from build123d import *

# Parameters (mm, degrees)
SKETCH1_R           = 1.5
SKETCH1_R_2         = 3.5
BOSS_EXTRUDE1_DEPTH = 5
FILLET1_R           = 3
FILLET2_R           = 8
SKETCH2_R           = 3.5
CUT_EXTRUDE1_DEPTH  = 2.5
CUT_EXTRUDE2_DEPTH  = 2


with BuildPart() as part:
    # Sketch1 → Boss-Extrude1 (new body)
    with BuildSketch(Plane(origin=(0, 0, 0), x_dir=(1, 0, 0), z_dir=(0, 1, 0))):
        Polygon((-34, -43.5), (-34, 43.5), (-97, 43.5), (-97, 20), (-112, 20), (-112, -20), (-97, -20), (-97, -43.5), align=None)
        with Locations(Location((-104.45, 0, 0), (0, 0, 270))):
            Circle(SKETCH1_R, mode=Mode.SUBTRACT)
        with Locations(Location((-43.45, 31, 0), (0, 0, 270))):
            Circle(SKETCH1_R_2, mode=Mode.SUBTRACT)
        with Locations(Location((-56.13, 25, 0), (0, 0, 270))):
            Circle(SKETCH1_R_2, mode=Mode.SUBTRACT)
        with Locations(Location((-40.45, 23.6, 0), (0, 0, 270))):
            Circle(SKETCH1_R, mode=Mode.SUBTRACT)
        with Locations(Location((-40.45, -23.6, 0), (0, 0, 270))):
            Circle(SKETCH1_R, mode=Mode.SUBTRACT)
        with Locations(Location((-56.13, -25, 0), (0, 0, 270))):
            Circle(SKETCH1_R_2, mode=Mode.SUBTRACT)
        with Locations(Location((-43.45, -31, 0), (0, 0, 270))):
            Circle(SKETCH1_R_2, mode=Mode.SUBTRACT)
        with Locations(Location((-39.5, 38, 0), (0, 0, 270))):
            Circle(SKETCH1_R, mode=Mode.SUBTRACT)
        with Locations(Location((-91.5, 38, 0), (0, 0, 270))):
            Circle(SKETCH1_R, mode=Mode.SUBTRACT)
        with Locations(Location((-91.5, -38, 0), (0, 0, 270))):
            Circle(SKETCH1_R, mode=Mode.SUBTRACT)
        with Locations(Location((-39.5, -38, 0), (0, 0, 270))):
            Circle(SKETCH1_R, mode=Mode.SUBTRACT)
    extrude(amount=BOSS_EXTRUDE1_DEPTH)

    # Fillet1
    fillet1_edges = [part.edges().sort_by_distance(p)[0] for p in [
        (-97, 2.5, 43.5),
        (-112, 2.5, 20),
        (-112, 2.5, -20),
        (-97, 2.5, -43.5),
        (-34, 2.5, -43.5),
        (-34, 2.5, 43.5),
    ]]
    fillet(fillet1_edges, radius=FILLET1_R)

    # Fillet2
    fillet2_edges = [part.edges().sort_by_distance(p)[0] for p in [
        (-97, 2.5, 20),
        (-97, 2.5, -20),
    ]]
    fillet(fillet2_edges, radius=FILLET2_R)

    # Sketch2 → Cut-Extrude1 (cut)
    with BuildSketch(Plane(origin=(0, 5, 0), x_dir=(1, 0, 0), z_dir=(0, 1, 0))):
        with Locations(Location((-40.45, -23.6, 0), (0, 0, 270))):
            Circle(SKETCH2_R)
        with Locations(Location((-40.45, 23.6, 0), (0, 0, 270))):
            Circle(SKETCH2_R)
        with Locations(Location((-104.45, 0, 0), (0, 0, 270))):
            Circle(SKETCH2_R)
    extrude(amount=-CUT_EXTRUDE1_DEPTH, mode=Mode.SUBTRACT)

    # Sketch3 → Cut-Extrude2 (cut)
    with BuildSketch(Plane.XZ):
        Polygon((-37.897853003, 35.225), (-36.295706006, 38), (-37.897853003, 40.775), (-41.102146997, 40.775), (-42.704293994, 38), (-41.102146997, 35.225), align=None)
        Polygon((-89.897853003, 35.225), (-88.295706006, 38), (-89.897853003, 40.775), (-93.102146997, 40.775), (-94.704293994, 38), (-93.102146997, 35.225), align=None)
        Polygon((-89.91228676, -35.25), (-93.08771324, -35.25), (-94.675426481, -38), (-93.08771324, -40.75), (-89.91228676, -40.75), (-88.324573519, -38), align=None)
        Polygon((-37.91228676, -40.75), (-36.324573519, -38), (-37.91228676, -35.25), (-41.08771324, -35.25), (-42.675426481, -38), (-41.08771324, -40.75), align=None)
    extrude(amount=-CUT_EXTRUDE2_DEPTH, mode=Mode.SUBTRACT)


solid = part.part
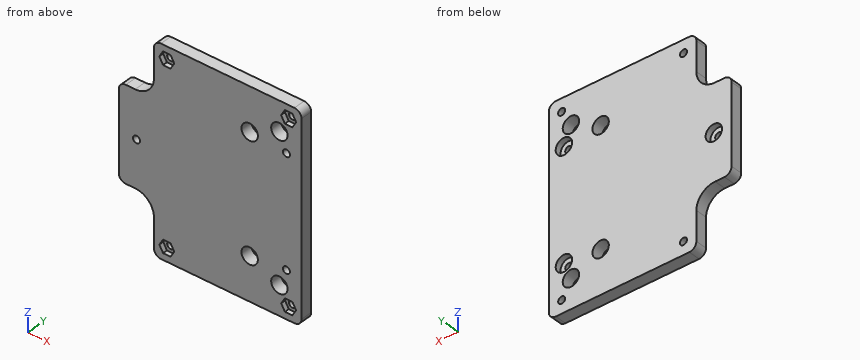
Work out the finished part from the listing and answer in its coordinate system (mm). Round coordinates to 2 decimals unless told otherwise and drop trailing zeros. Write each loop counter-clockwise with the first axis right and the second up, starting at its lowest first coordinate (ties: lowest second). Pieces come first, ordered by that corner, then holes. Notation, with made-up numbers: M 58,-11 L 117,-11 A24 ccw 117,4 Z; hole C -26.5,65 d11. An arc over 180 degrees is marked long. Use a Markdown table: item, result.
1) The part is cut by section C-C on y = 3.85. State how many separate pieces and enclosed holes the cut face has, plus the area to 3 significant figures.
Taken from the geometry:
| item | result |
|---|---|
| separate pieces | 1 |
| enclosed holes | 11 |
| area | 5,800 mm2 |
2) The part is cut by section A-A on x = -56.13. Give the vertices of the cut face in (y, z).
Taken from the geometry:
| item | result |
|---|---|
| outline | M 0,-43.5 L 5,-43.5 L 5,-28.5 L 0,-28.5 Z; M 0,-21.5 L 5,-21.5 L 5,21.5 L 0,21.5 Z; M 0,28.5 L 5,28.5 L 5,43.5 L 0,43.5 Z |
3) Consider line 1 (X direction, y = 3.6, z = -38); line 2 (X direction, y = 2.8, z = 37); line 3 (Z direction, x = -42, y = 3.7). Determine where each line is inside the solid, lowest interval first. Write a range as [from, to].
Taken from the geometry:
| item | result |
|---|---|
| line 1 | x = [-97, -93], [-90, -41], [-38, -34] |
| line 2 | x = [-97, -92.62], [-90.38, -40.62], [-38.38, -34] |
| line 3 | z = [-43.5, -34.19], [-27.81, -26.74], [-20.46, 20.46], [26.74, 27.81], [34.19, 43.5] |
4) The part is cut by section B-B on z = 0. Give the vertices of the cut face in (x, y), plus the area to 3 significant figures.
Taken from the geometry:
| item | result |
|---|---|
| outline | M -112,0 L -105.95,0 L -105.95,2.5 L -107.95,2.5 L -107.95,5 L -112,5 Z; M -102.95,0 L -34,0 L -34,5 L -100.95,5 L -100.95,2.5 L -102.95,2.5 Z |
| area | 365 mm2 |
5) Flat-ended cylindrical pins translate along their axes: pin 1 (6 mm diameter, centred on x = -40, z = 37, fed in from -Y); pin 2 (1.2 mm diameter, centred on x = -106.5, y = 2.5, fed in from +Z); pin 3 (2 mm diameter, centred on x = -103.5, z = -1, fed in from +Y). Find the tip coordinate at first contact, or state that the pin passes through.
Taken from the geometry:
| item | result |
|---|---|
| pin 1 | stops at y = 0 |
| pin 2 | stops at z = 20 |
| pin 3 | stops at y = 2.5 |
6) The part is cut by section D-D on z = 23.6. Give the vertices of the cut face in (x, y), plus the area to 3 significant figures.
Taken from the geometry:
| item | result |
|---|---|
| outline | M -98.32,0 L -59.34,0 L -59.34,5 L -98.32,5 Z; M -52.92,0 L -41.95,0 L -41.95,2.5 L -43.95,2.5 L -43.95,5 L -52.92,5 Z; M -38.95,0 L -34,0 L -34,5 L -36.95,5 L -36.95,2.5 L -38.95,2.5 Z |
| area | 265 mm2 |
